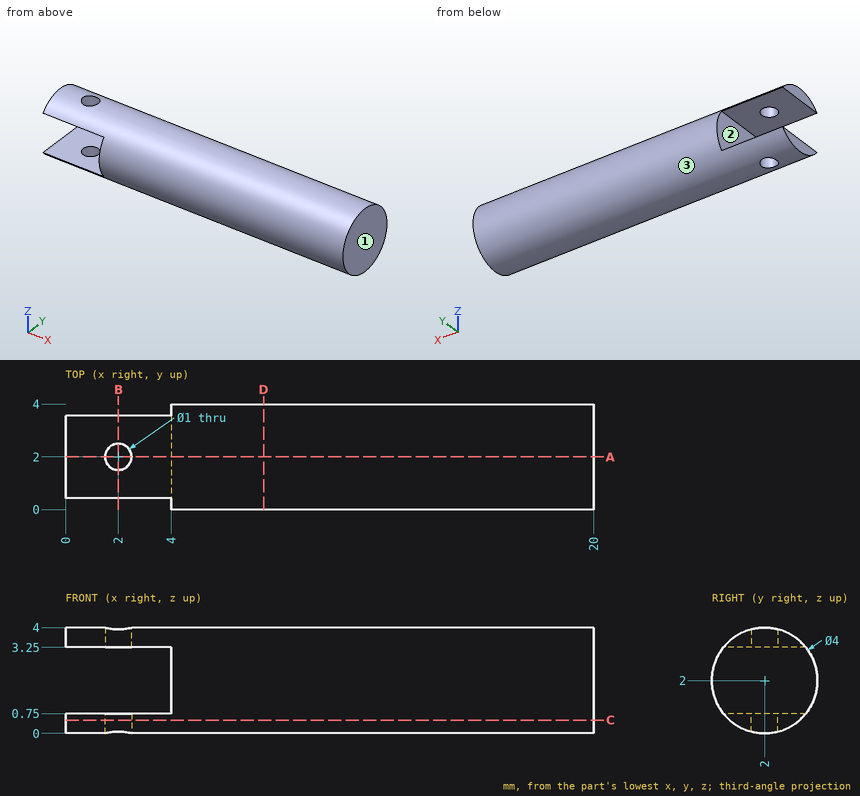
Could you check a few things on this drawing? It's one solid part, dimensions in mm from its lowest x, y, z. Give positions to 0.01 mm unless a question says otherwise; leave off trailing zeros. Order: outer loops, then holes, each group sorted by start corner. A loop starts at its lowest first (then second) coordinate and runs counter-clockwise, first axis right, second up. Notation, with made-up numbers: (7.25, 65.5) -> (17.25, 65.5) arc R16 cw to (17.25, 76.5) -> close; hole circle Ø3 at (24, 32.5). An arc over 180 degrees is marked (long way). Use CSV: the item, a comma, the result in double quotes. Start each with the question number.
Item 1: Thinking about a two-plate mould opening in Z: for the marked faces 1, 2 and 3, which applies, pulls with the +Z half, pulls with the -Z half, needs draft (parallel to the pull), parting line crosses it, or undercut?
Item 2: Suppose I cut it at C-C (z = 0.5). List the corners of the cut face in (x, y) for me, and give its area (3 significant figures).
Item 3: I'm going to push a flat-ended pin straight in: P1, Ø0.8, axis at y = 1, z = 2, coming from the -X side. Where does the tip first touch, or does it pass through?
Item 4: If I drill on probe 1 along Y at (x, z) = (6.5, 0.75); probe 2 along X at (y, z) = (0.2, 1.6); probe 3 along Z at (x, y) = (3, 0.7), over which ranges is the centre line in solid material (lowest first)? Write a range as [from, to].
Item 5: Suppose I cut it at B-B (x = 2). List the corners of the cut face in (y, z) for me.
Item 6: Suppose I cut it at A-A (y = 2). List the corners of the cut face in (x, z) for me.
Item 7: Suppose I cut it at D-D (x = 7.5). List the corners of the cut face in (y, z) for me, and give its area (3 significant figures).
Answer block:
1,face 1,"needs draft"
1,face 2,"undercut"
1,face 3,"parting line crosses it"
2,outline,"(0, 0.68) -> (20, 0.68) -> (20, 3.32) -> (0, 3.32) -> close; hole circle Ø1 at (2, 2)"
2,area,"52.1 mm^2"
3,P1,"stops at x = 4"
4,probe 1,"y = [0.44, 3.56]"
4,probe 2,"x = [4, 20]"
4,probe 3,"z = [0.48, 0.75], [3.25, 3.52]"
5,outline,"(0.44, 0.75) arc R2 ccw to (1.5, 0.06) -> (1.5, 0.75) -> close; (0.44, 3.25) -> (1.5, 3.25) -> (1.5, 3.94) arc R2 ccw to start; (2.5, 0.06) arc R2 ccw to (3.56, 0.75) -> (2.5, 0.75) -> close; (2.5, 3.25) -> (3.56, 3.25) arc R2 ccw to (2.5, 3.94) -> close"
6,outline,"(0, 0) -> (1.5, 0) -> (1.5, 0.75) -> (0, 0.75) -> close; (0, 3.25) -> (1.5, 3.25) -> (1.5, 4) -> (0, 4) -> close; (2.5, 0) -> (20, 0) -> (20, 4) -> (2.5, 4) -> (2.5, 3.25) -> (4, 3.25) -> (4, 0.75) -> (2.5, 0.75) -> close"
7,outline,"circle Ø4 at (2, 2)"
7,area,"12.6 mm^2"
